Here's how the part is built. I have some questions about the finished solid (model axes, mm). Face numbers are marked on the shaded views. Give positions to 0.01 mm unless a question says otherwise; leave off trailing zeros. Write each loop counter-clockwise with the first axis right and the second up, starting at its lowest first coordinate (ties: lowest second). Pieces come first, ordered by that corner, then holes. Notation, with made-up numbers: (-9, 24.25) - (11, 24.25) arc R24 ccw to (11, 54.25) - close; hole circle Ø5 at (-24, 19). An arc over 180 degrees is marked (long way). Write each question's results on one line, items separated by ' | '. Start each with the question number.
Item 1: Suppose I cut it at B-B on z = 250. List the corners of the cut face in (x, y) for me (1 decimal).
Item 2: We'd pull the mould along Y, two halves only. Please class the marked faces 1, 2 and 3: +Y half, -Y half, draft (parallel to the pull), parting line (faces both ways), or undercut.
Item 3: Will these pins go through, and if not, where does the flat tip stop? P1, Ø4, axis at y = -18.5, z = 39.5, coming from the -X side; P2, Ø8, axis at x = -8.5, z = 236, coming from the +Y side; P3, Ø2, axis at x = -19.5, y = 17, coming from the +Z side.
Item 4: Please list where these lines run through material, in increasing order: line 1 along Y through (x, z) = (17.5, 146); line 2 along X through (y, z) = (19, 258); line 3 along Z through (x, y) = (-5, -22).
Item 5: Suppose I cut it at A-A on y = 0. List the corners of the cut face in (x, z) for me (1 decimal).
Item 6: Suppose I cut it at C-C on x = 0. List the corners of the cut face in (y, z) for me (1 decimal), then the cut area to 3 significant figures.
```python
from build123d import *

# Parameters (mm, degrees)
F0_R      = 20.6375
F0_R_2    = 3.9624
F1_DEPTH  = 279.4
F2_W      = 50.8
F2_H      = 50.8
F3_DEPTH  = 25.4
F4_W      = 50.8
F4_H      = 50.8
F5_DEPTH  = 50.8
F6_R      = 3.302
F7_DEPTH  = 17.78
F8_R      = 3.302
F9_DEPTH  = 17.78
F10_R     = 15.875
F11_DEPTH = 3.175
F12_R     = 5.715
F13_DEPTH = 12.7


with BuildPart() as f1:
    # F0 (on Top) → F1 (new body)
    with BuildSketch(Plane.XY):
        Circle(F0_R)
        with Locations((-17.9451, 17.9451)):
            Circle(F0_R_2)
        with Locations((17.9451, 17.9451)):
            Circle(F0_R_2)
        with Locations((17.9451, -17.9451)):
            Circle(F0_R_2)
        with Locations((-17.9451, -17.9451)):
            Circle(F0_R_2)
    extrude(amount=F1_DEPTH)

    # F2 (on face) → F3 (join)
    with BuildSketch(Plane.XY.offset(279.4)):
        Rectangle(F2_W, F2_H)
    extrude(amount=F3_DEPTH)

    # F4 (on face) → F5 (join)
    with BuildSketch(Plane(origin=(0, 0, 0), x_dir=(1, 0, 0), z_dir=(0, 0, -1))):
        Rectangle(F4_W, F4_H)
    extrude(amount=F5_DEPTH)

    # F6 (on face) → F7 (cut)
    with BuildSketch(Plane(origin=(0, 0, -50.8), x_dir=(1, 0, 0), z_dir=(0, 0, -1))):
        with Locations((-17.9451, 17.9451)):
            Circle(F6_R)
        with Locations((17.9451, 17.9451)):
            Circle(F6_R)
        with Locations((17.9451, -17.9451)):
            Circle(F6_R)
        with Locations((-17.9451, -17.9451)):
            Circle(F6_R)
    extrude(amount=-F7_DEPTH, mode=Mode.SUBTRACT)

    # F8 (on face) → F9 (cut)
    with BuildSketch(Plane.XY.offset(304.8)):
        with Locations((17.9451, -17.9451)):
            Circle(F8_R)
        with Locations((-17.9451, -17.9451)):
            Circle(F8_R)
        with Locations((17.9451, 17.9451)):
            Circle(F8_R)
        with Locations((-17.9451, 17.9451)):
            Circle(F8_R)
    extrude(amount=-F9_DEPTH, mode=Mode.SUBTRACT)

    # F10 (on face) → F11 (cut)
    with BuildSketch(Plane(origin=(0, 0, -50.8), x_dir=(1, 0, 0), z_dir=(0, 0, -1))):
        Circle(F10_R)
    extrude(amount=-F11_DEPTH, mode=Mode.SUBTRACT)

    # F12 (on face) → F13 (cut)
    with BuildSketch(Plane(origin=(0, 25.4, 0), x_dir=(-1, 0, 0), z_dir=(0, 1, 0))):
        with Locations((0, -16.51)):
            Circle(F12_R)
        with Locations((0, 295.148)):
            Circle(F12_R)
    extrude(amount=-F13_DEPTH, mode=Mode.SUBTRACT)


solid = f1.part
```
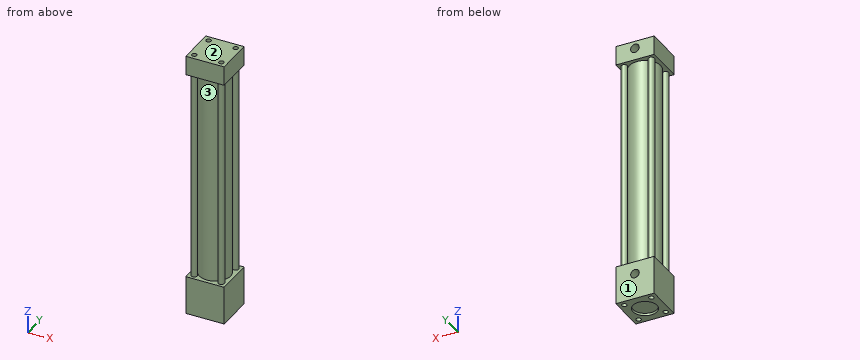
Checked values:
1) outline: circle Ø7.9 at (-17.9, -17.9); circle Ø7.9 at (-17.9, 17.9); circle Ø41.3 at (0, 0); circle Ø7.9 at (17.9, -17.9); circle Ø7.9 at (17.9, 17.9)
2) face 1: +Y half | face 2: draft | face 3: undercut
3) P1: stops at x = -21.91 | P2: stops at y = 20.14 | P3: stops at z = 287.02
4) line 1: y = -21.88 to -14.01, -10.94 to 10.94, 14.01 to 21.88 | line 2: x = -21.76 to -14.13, -8.06 to 8.06, 14.13 to 21.76 | line 3: z = -50.8 to 0, 279.4 to 304.8
5) outline: (-25.4, -50.8) - (-15.9, -50.8) - (-15.9, -47.6) - (15.9, -47.6) - (15.9, -50.8) - (25.4, -50.8) - (25.4, 0) - (20.6, 0) - (20.6, 279.4) - (25.4, 279.4) - (25.4, 304.8) - (-25.4, 304.8) - (-25.4, 279.4) - (-20.6, 279.4) - (-20.6, 0) - (-25.4, 0) - close
6) outline: (-25.4, -50.8) - (-15.9, -50.8) - (-15.9, -47.6) - (15.9, -47.6) - (15.9, -50.8) - (25.4, -50.8) - (25.4, -22.2) - (12.7, -22.2) - (12.7, -10.8) - (25.4, -10.8) - (25.4, 0) - (20.6, 0) - (20.6, 279.4) - (25.4, 279.4) - (25.4, 289.4) - (12.7, 289.4) - (12.7, 300.9) - (25.4, 300.9) - (25.4, 304.8) - (-25.4, 304.8) - (-25.4, 279.4) - (-20.6, 279.4) - (-20.6, 0) - (-25.4, 0) - close | area: 15,000 mm^2
